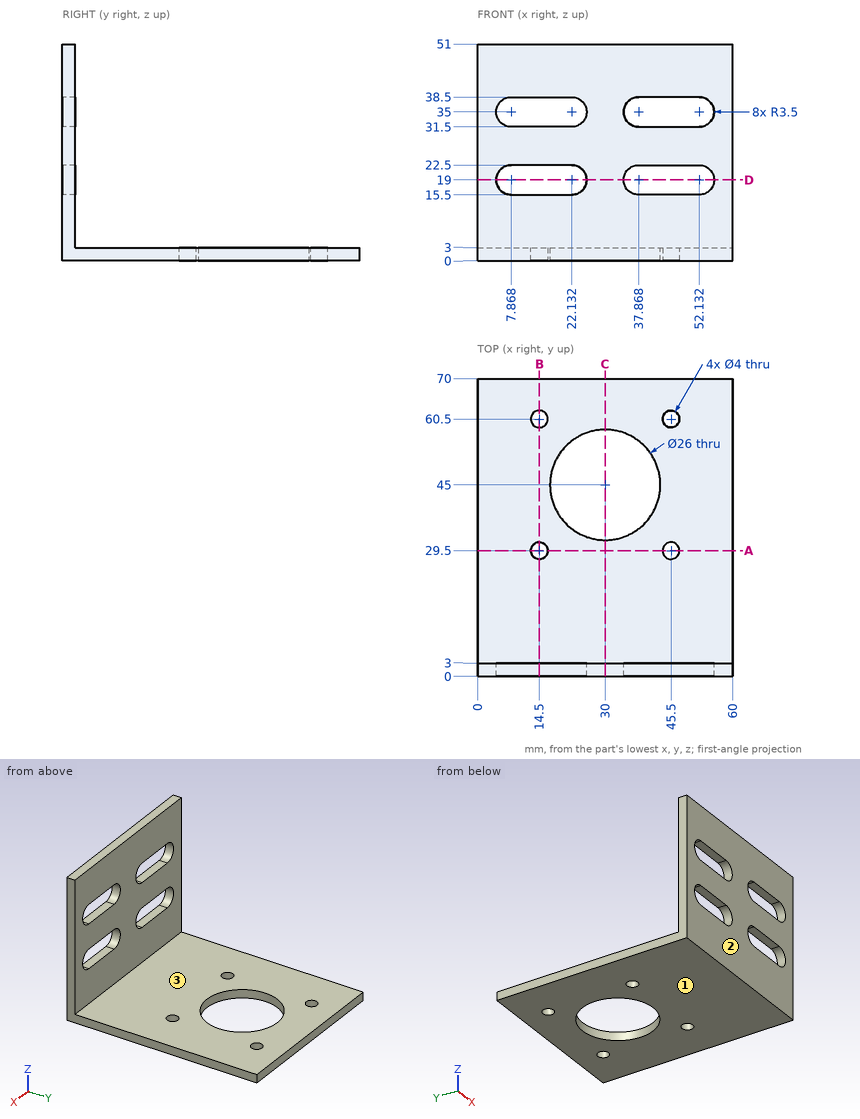
Job drawing, mm, ordinate dimensions from the low corner. One solid piece. Round coordinates to 2 decimals unless told otherwise and drop trailing zeros. Loops run counter-clockwise (first coordinate to the right, second up) from the corner with the lowest first, then second, coordinate; pieces in that order, holes last.
Item 1: Drill centre lines: line 1 (Y direction, x = 45.5, z = 0.8); line 2 (Z direction, x = 48, y = 12.5); line 3 (Y direction, x = 45, z = 1). Where is each one in solid material? Low to high.
Item 2: Cut at A-A, the plane y = 29.5. Give the cut face in (x, z), then the cut area to 3 significant figures.
Item 3: Cut at D-D, the plane z = 19. Give the cut face in (x, y).
Item 4: Mould opens along Z. For the marked faces 1, 2 and 3 say: +Z half, -Z half, draft (parallel to the pull), parting line (faces both ways), or undercut.
Item 5: Cut at B-B, the plane x = 14.5. Give the cut face in (y, z), then the cut area to 3 significant figures.
Item 6: Drop flat-ended pins along their axis: P1, Ø4.5, axis at x = 45.5, y = 29.5, coming from the +Z side; P2, Ø6, axis at x = 10, z = 24, coming from the +Y side. Give the stop position or say it passes through.
Item 7: Cut at C-C, the plane x = 30. Give the cut face in (y, z).
A:
1. line 1: y = 0 to 27.5, 31.5 to 58.5, 62.5 to 70
1. line 2: z = 0 to 3
1. line 3: y = 0 to 27.56, 31.44 to 58.56, 62.44 to 70
2. outline: (0, 0) - (12.5, 0) - (12.5, 3) - (0, 3) - close; (16.5, 0) - (43.5, 0) - (43.5, 3) - (16.5, 3) - close; (47.5, 0) - (60, 0) - (60, 3) - (47.5, 3) - close
2. area: 156 mm2
3. outline: (0, 0) - (4.37, 0) - (4.37, 3) - (0, 3) - close; (25.63, 0) - (34.37, 0) - (34.37, 3) - (25.63, 3) - close; (55.63, 0) - (60, 0) - (60, 3) - (55.63, 3) - close
4. face 1: -Z half
4. face 2: draft
4. face 3: +Z half
5. outline: (0, 0) - (27.5, 0) - (27.5, 3) - (3, 3) - (3, 15.5) - (0, 15.5) - close; (0, 22.5) - (3, 22.5) - (3, 31.5) - (0, 31.5) - close; (0, 38.5) - (3, 38.5) - (3, 51) - (0, 51) - close; (31.5, 0) - (58.5, 0) - (58.5, 3) - (31.5, 3) - close; (62.5, 0) - (70, 0) - (70, 3) - (62.5, 3) - close
5. area: 288 mm2
6. P1: stops at z = 3
6. P2: stops at y = 3
7. outline: (0, 0) - (32, 0) - (32, 3) - (3, 3) - (3, 51) - (0, 51) - close; (58, 0) - (70, 0) - (70, 3) - (58, 3) - close
